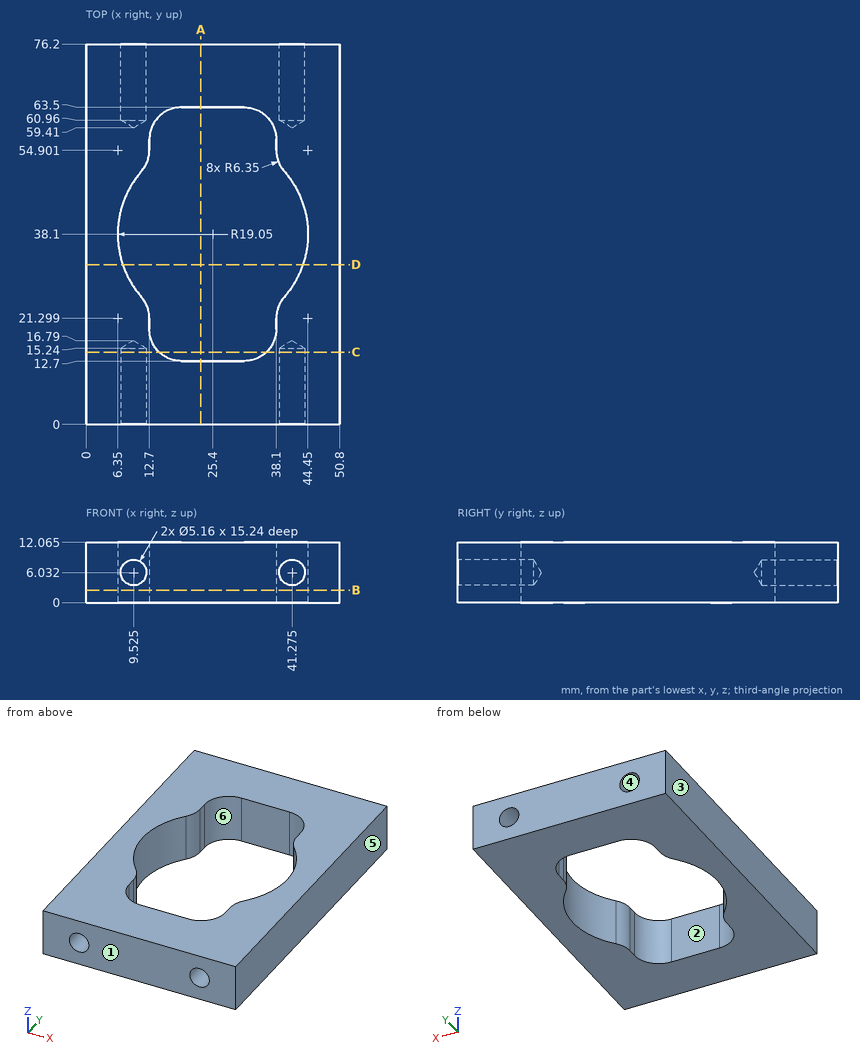
Answer from the drawing. Dimensions are ordinates in mm from the lowest x, y and z of the part. A direction names the side the tool comes from. Coordinates: 2 decimals unless noted, no trailing zeros. Order: outer loops, then holes, each group sorted by start corner. A loop starts at its lowest first (then second) coordinate and runs counter-clockwise, first axis right, second up. Notation, with made-up numbers: (38.5, 6.25) -> (96.5, 6.25) arc R13 ccw to (96.5, 16.25) -> close; hole circle Ø4 at (20.5, 54.25). An arc over 180 degrees is marked (long way). Answer as a JSON object with one key per item and string values.
1) A cutting plane is placed at D-D, the plane y = 32. Determine the outline of the cut face in (x, z) (1 decimal).
Model answer:
{"outline": "(0, 0) -> (7.4, 0) -> (7.4, 12.1) -> (0, 12.1) -> close; (43.4, 0) -> (50.8, 0) -> (50.8, 12.1) -> (43.4, 12.1) -> close"}
2) Consider line 1 along X through (y, z) = (65, 6) (1 decimal); line 2 along Y through (x, z) = (24, 6); line 3 along X through (y, z) = (11.5, 5.5). Determine where each line is inside the solid, lowest interval first. Write a range as from..to.
Model answer:
{"line 1": "x = 0..6.9, 12.1..38.7, 43.9..50.8", "line 2": "y = 0..12.7, 63.5..76.2", "line 3": "x = 0..7, 12.05..38.75, 43.8..50.8"}
3) A cutting plane is placed at C-C, the plane y = 14.5. Determine the outline of the cut face in (x, z) (1 decimal), plus the area to 3 significant figures.
Model answer:
{"outline": "(0, 0) -> (14.6, 0) -> (14.6, 12.1) -> (0, 12.1) -> close; (36.2, 0) -> (50.8, 0) -> (50.8, 12.1) -> (36.2, 12.1) -> close; hole circle Ø5.2 at (9.5, 6); hole circle Ø5.2 at (41.3, 6)", "area": "311 mm²"}
4) A cutting plane is placed at B-B, the plane z = 2.5. Determine the outline of the cut face in (x, y), plus the area to 3 significant figures.
Model answer:
{"outline": "(0, 0) -> (50.8, 0) -> (50.8, 76.2) -> (0, 76.2) -> close; hole (11.11, 25.5) arc R6.35 cw to (12.7, 21.3) -> (12.7, 19.05) arc R6.35 ccw to (19.05, 12.7) -> (31.75, 12.7) arc R6.35 ccw to (38.1, 19.05) -> (38.1, 21.3) arc R6.35 cw to (39.69, 25.5) arc R19.05 ccw to (39.69, 50.7) arc R6.35 cw to (38.1, 54.9) -> (38.1, 57.15) arc R6.35 ccw to (31.75, 63.5) -> (19.05, 63.5) arc R6.35 ccw to (12.7, 57.15) -> (12.7, 54.9) arc R6.35 cw to (11.11, 50.7) arc R19.05 ccw to start", "area": "2,360 mm²"}
5) Each of these flat-tipped pins is pushed along its axis until it touches: pin 1 (4.5 mm diameter, centred on x = 41.28, z = 6.03, fed in from -Y) (1 decimal); pin 2 (2.5 mm diameter, centred on y = 20, z = 5, fed in from -X); pin 3 (4 mm diameter, centred on x = 41.28, z = 6.03, fed in from +Y) (1 decimal); pin 4 (4 mm diameter, centred on x = 9.52, z = 6.03, fed in from -Y) (1 decimal). Where does it stop, or does it pass through?
Model answer:
{"pin 1": "stops at y = 15.4", "pin 2": "stops at x = 0", "pin 3": "stops at y = 60.6", "pin 4": "stops at y = 15.6"}
6) A tool of negligible diameter and unlimited length cuts with its end or side. For the marked faces 4, 5 and 6, from which of +Z, -Z, +X, -X, +Y, -Y can it reach the whole face along a straight path? Write none if from no direction.
Model answer:
{"face 4": "+Y", "face 5": "+Z, -Z, +X, +Y, -Y", "face 6": "+Z, -Z"}
7) The mould has two halves that part along X. Classify the marked faces 1, 2 and 3: released by +X, released by -X, zero draft, split by the parting line, or undercut.
Model answer:
{"face 1": "zero draft", "face 2": "undercut", "face 3": "released by -X"}
8) A cutting plane is placed at A-A, the plane x = 23. Determine the outline of the cut face in (y, z) (1 decimal).
Model answer:
{"outline": "(0, 0) -> (12.7, 0) -> (12.7, 12.1) -> (0, 12.1) -> close; (63.5, 0) -> (76.2, 0) -> (76.2, 12.1) -> (63.5, 12.1) -> close"}
